from build123d import *

# Parameters (mm, degrees)
F0_W     = 101.6
F0_H     = 76.2
F1_DEPTH = 38.1
F2_R     = 25.4
F3_DEPTH = 19.05
F4_R     = 19.05
F5_DEPTH = 19.05
F6_R     = 5.08


with BuildPart() as f1:
    # F0 (on Top) → F1 (new body)
    with BuildSketch(Plane.XY):
        with Locations((15.432196, -3.358119)):
            Rectangle(F0_W, F0_H)
    extrude(amount=F1_DEPTH)

    # F2 (on face) → F3 (join)
    with BuildSketch(Plane.XY.offset(38.1)):
        with Locations((14.508507, 0)):
            Circle(F2_R)
    extrude(amount=F3_DEPTH)

    # F4 (on face) → F5 (join)
    with BuildSketch(Plane.XY.offset(57.15)):
        with Locations((14.508507, 0)):
            Circle(F4_R)
    extrude(amount=F5_DEPTH)

    # F6
    f6_edges = [f1.edges().sort_by_distance(p)[0] for p in [
        (15.432196, 34.741881, 38.1),
        (66.232196, 34.741881, 19.05),
        (15.432196, 34.741881, 0),
        (-35.367804, 34.741881, 19.05),
        (66.232196, -3.358119, 38.1),
        (66.232196, -3.358119, 0),
        (66.232196, -41.458119, 19.05),
        (15.432196, -41.458119, 38.1),
        (-35.367804, -3.358119, 38.1),
        (15.432196, -41.458119, 0),
        (-35.367804, -3.358119, 0),
        (-35.367804, -41.458119, 19.05),
    ]]
    fillet(f6_edges, radius=F6_R)


solid = f1.part
Model file for the job. Use its own axes, mm. A direction names the side the tool comes from. Round coordinates to 2 decimals unless told otherwise and drop trailing zeros. Loops run counter-clockwise (first coordinate to the right, second up) from the corner with the lowest first, then second, coordinate; pieces in that order, holes last.
1. Band-saw the part on A-A, the plane y = 0. List the corners of the cut face in (x, z), and give its area (3 significant figures).
Check values:
outline: (-35.37, 5.08) arc R5.08 ccw to (-30.29, 0) - (61.15, 0) arc R5.08 ccw to (66.23, 5.08) - (66.23, 33.02) arc R5.08 ccw to (61.15, 38.1) - (39.91, 38.1) - (39.91, 57.15) - (33.56, 57.15) - (33.56, 76.2) - (-4.54, 76.2) - (-4.54, 57.15) - (-10.89, 57.15) - (-10.89, 38.1) - (-30.29, 38.1) arc R5.08 ccw to (-35.37, 33.02) - close
area: 5,540 mm2
2. Tool access for faces 1 (the flat face through (18, 19, 57.15)), 2 (the cylindrical face through (16.072, 33.293, 36.572)): list every direction of +Z, -Z, +X, -X, +Y, -Y with a clear straight run to the whole face (end or side of a thin tool).
Check values:
face 1: +Z
face 2: +Z, +X, -X, +Y
3. Drop flat-ended pins along their axis: P1, Ø6, axis at x = -11, y = -14.5, coming from the +Z side; P2, Ø10, axis at x = -16.5, z = 57, coming from the +Y side; P3, Ø4, axis at x = 24, y = -23.5, coming from the +Z side. Give the stop position or say it passes through.
Check values:
P1: stops at z = 38.1
P2: passes through
P3: stops at z = 57.15
4. Band-saw the part on D-D, the plane z = 66. List the corners of the cut face in (x, y).
Check values:
outline: circle Ø38.1 at (14.51, 0)
5. Band-saw the part on B-B, the plane x = 50. List the corners of the cut face in (y, z).
Check values:
outline: (-41.46, 5.08) arc R5.08 ccw to (-36.38, 0) - (29.66, 0) arc R5.08 ccw to (34.74, 5.08) - (34.74, 33.02) arc R5.08 ccw to (29.66, 38.1) - (-36.38, 38.1) arc R5.08 ccw to (-41.46, 33.02) - close
6. Band-saw the part on C-C, the plane y = -33.5. List the corners of the cut face in (x, z).
Check values:
outline: (-35.37, 5.08) arc R5.08 ccw to (-30.29, 0) - (61.15, 0) arc R5.08 ccw to (66.23, 5.08) - (66.23, 33.02) arc R5.08 ccw to (61.15, 38.1) - (-30.29, 38.1) arc R5.08 ccw to (-35.37, 33.02) - close
7. Wall check: probe 1 along X at (y, z) = (15, 5); probe 2 along Z at (x, y) = (51, -18.5); probe 3 along Z at (x, y) = (-9, 5). Give the ranges that are in metal, low to high.
Check values:
probe 1: x = -35.37 to 66.23
probe 2: z = 0 to 38.1
probe 3: z = 0 to 57.15
